Verification items for the finished model (mm, model axes). A direction names the side the tool comes from. Round coordinates to 2 decimals unless told otherwise and drop trailing zeros. Write each loop counter-clockwise with the first axis right and the second up, starting at its lowest first coordinate (ties: lowest second). Pieces come first, ordered by that corner, then holes.
from build123d import *

# Parameters (mm, degrees)
F0_R          = 44.45
F1_DEPTH      = 1000
F0_R_2        = 96
F0_R_3        = 92.5
F2_R          = 7.5
F2_R_2        = 6.5
F3_DEPTH      = 15
F4_R          = 96
F5_DEPTH      = 25
F5_DEPTH_BACK = 25
F6_R          = 7.5
F6_R_2        = 6.5
F7_DEPTH      = 15


with BuildPart() as f1:
    # F0 (on Top) → F1 (new body)
    with BuildSketch(Plane.XY):
        with Locations((-32.7036886299, -32.7036886299)):
            Circle(F0_R)
    extrude(amount=F1_DEPTH)



with BuildPart() as f1b:
    # F0 (on Top) → F1, piece 2 (new body)
    with BuildSketch(Plane.XY):
        with Locations((32.7036886299, 32.7036886299)):
            Circle(F0_R)
    extrude(amount=F1_DEPTH)

    # F2 (on face) → F3 (join)
    with BuildSketch(Plane(origin=(0, 0, 0), x_dir=(1, 0, 0), z_dir=(0, 0, -1))):
        with Locations((32.7036886299, -32.7036886299)):
            Circle(F2_R)
        with Locations((32.7036886299, -32.7036886299)):
            Circle(F2_R_2, mode=Mode.SUBTRACT)
    extrude(amount=F3_DEPTH)


with BuildPart() as f1c:
    # F0 (on Top) → F1, piece 3 (new body)
    with BuildSketch(Plane.XY):
        Circle(F0_R_2)
        Circle(F0_R_3, mode=Mode.SUBTRACT)
    extrude(amount=F1_DEPTH)


with BuildPart() as f1_1:
    add(f1.part)

    add(f1b.part)  # F5 merges F1b

    add(f1c.part)  # F5 merges F1c
    # F4 (on face) → F5 (join, two sides)
    with BuildSketch(Plane.XY.offset(1000)) as f5_sk:
        Circle(F4_R)
    extrude(amount=F5_DEPTH)
    extrude(f5_sk.sketch, amount=-F5_DEPTH_BACK)

    # F6 (on face) → F7 (join)
    with BuildSketch(Plane(origin=(0, 0, 0), x_dir=(1, 0, 0), z_dir=(0, 0, -1))):
        with Locations((-32.7036886299, 32.7036886299)):
            Circle(F6_R)
        with Locations((-32.7036886299, 32.7036886299)):
            Circle(F6_R_2, mode=Mode.SUBTRACT)
    extrude(amount=F7_DEPTH)


solid = f1_1.part
Q1. Sectioned sample at C-C (x = -53). Enter the section's corners in (y, z), plus the area to 3 significant figures.
Recorded:
outline: (-80.04, 0) - (-75.81, 0) - (-75.81, 975) - (-72.25, 975) - (-72.25, 0) - (6.84, 0) - (6.84, 975) - (75.81, 975) - (75.81, 0) - (80.04, 0) - (80.04, 1025) - (-80.04, 1025) - close
area: 93,400 mm2
Q2. Release check for a two-part mould opening along Y. For faces 1 (the flat face through (-23, -32, 0)), 2 (the cylindrical face through (23.07, -10.69, 480.68)) record: released by +Y, released by -Y, zero draft, split by the parting line, or undercut.
Recorded:
face 1: zero draft
face 2: undercut
Q3. Sectioned sample at B-B (z = 622). Enter the section's corners in (x, y).
Recorded:
outline: circle Ø192 at (0, 0); circle Ø88.9 at (-32.7, -32.7); circle Ø88.9 at (32.7, 32.7); hole circle Ø185 at (0, 0)
Q4. Sectioned sample at A-A (y = 0). Enter the section's corners in (x, z).
Recorded:
outline: (-96, 0) - (-92.5, 0) - (-92.5, 975) - (-62.81, 975) - (-62.81, 0) - (-2.6, 0) - (-2.6, 975) - (2.6, 975) - (2.6, 0) - (62.81, 0) - (62.81, 975) - (92.5, 975) - (92.5, 0) - (96, 0) - (96, 1025) - (-96, 1025) - close
Q5. Material ranges on line 1 along X through (y, z) = (28, 50); line 2 along Y through (x, z) = (51, 731.5); line 3 along Y through (x, z) = (-63.5, 888), recorded low to high.
Recorded:
line 1: x = -91.83 to -88.16, -11.5 to 76.9, 88.16 to 91.83
line 2: y = -81.33 to -77.17, -7.81 to 73.21, 77.17 to 81.33
line 3: y = -72 to -67.26, -64.76 to -0.65, 67.26 to 72
Q6. Tool access check on faces 3 (the cylindrical face through (49.727, 77.996, 480.675)), 4 (the flat face through (-1, 1, 1025)). Record the directions out of +Z, -Z, +X, -X, +Y, -Y that give a thin tool (end or side, any length) a straight path to the whole face; none if there is none.
Recorded:
face 3: -Z
face 4: +Z, +X, -X, +Y, -Y
Q7. Depth check by flat-ended pin: P1, Ø11.5, axis at x = -32.7, y = -32.7, coming from the -Z side; P2, Ø3, axis at x = -25, z = 697, coming from the +Y side; P3, Ø12, axis at x = -18, z = 404.5, coming from the -Y side. Enter the tip coordinate at first touch or a pass-through.
Recorded:
P1: stops at z = 0
P2: stops at y = 93.08
P3: stops at y = -95.25
